from build123d import *

# Parameters (mm, degrees)
F1_DEPTH       = 30
F3_D           = 12.6
F3_CBORE_D     = 19.25
F3_CBORE_DEPTH = 12
F5_DEPTH       = 20
F7_DEPTH       = 10
F9_T1_DEPTH    = 80.6698729811
F9_T3_DEPTH    = 37.5
F9_T5_DEPTH    = 30
F9_T7_DEPTH    = 81.3397459622
F9_T9_DEPTH    = 40
F9_T12_ANGLE   = 90
F9_T14_ANGLE   = 90
F9_T16_ANGLE   = 117.3060073295
F9_T18_ANGLE   = 90
F9_T20_ANGLE   = 180
F9_T22_ANGLE   = 180
F10_DEPTH      = 20.001


# Not quite as in the source:
# - a fillet or chamfer that OpenCascade refuses, or shapes differently, is made with other operations: its cross-section is extruded or revolved along the edge and cut away or added


with BuildPart() as f1:
    # F0 (on Top) → F1 (new body)
    with BuildSketch(Plane.XY):
        with BuildLine():
            Line((0, -30), (0, 0))
            Line((0, 0), (30, 30))
            Line((30, 30), (40, 30))
            ThreePointArc((40, 30), (47.0710678119, 32.9289321881), (50, 40))
            Line((50, 40), (50, 50))
            ThreePointArc((50, 50), (47.0710678119, 57.0710678119), (40, 60))
            Line((40, 60), (-45, 60))
            ThreePointArc((-45, 60), (-48.6602540378, 56.3397459622), (-50, 51.3397459622))
            Line((-50, 51.3397459622), (-50, -30))
            ThreePointArc((-50, -30), (-47.0710678119, -37.0710678119), (-40, -40))
            Line((-40, -40), (-10, -40))
            ThreePointArc((-10, -40), (-2.9289321881, -37.0710678119), (0, -30))
        make_face()
    extrude(amount=F1_DEPTH)

    # F3 (through all)
    with Locations(Plane.XY.offset(30)):
        with Locations((35, 45)):
            CounterBoreHole(F3_D / 2, F3_CBORE_D / 2, F3_CBORE_DEPTH)

    # F4 (on face) → F5 (cut)
    with BuildSketch(Plane.XY.offset(30)):
        with BuildLine():
            Line((-10, 55.6698729811), (-42.5, 55.6698729811))
            ThreePointArc((-42.5, 55.6698729811), (-44.3301270189, 53.8397459622), (-45, 51.3397459622))
            Line((-45, 51.3397459622), (-45, -30))
            ThreePointArc((-45, -30), (-43.5355339059, -33.5355339059), (-40, -35))
            Line((-40, -35), (-10, -35))
            ThreePointArc((-10, -35), (-6.4644660941, -33.5355339059), (-5, -30))
            Line((-5, -30), (-5, 50.6698729811))
            ThreePointArc((-5, 50.6698729811), (-6.4644660941, 54.205406887), (-10, 55.6698729811))
        make_face()
    extrude(amount=-F5_DEPTH, mode=Mode.SUBTRACT)

    # F6 (on face) → F7 (join)
    with BuildSketch(Plane.XY.offset(10)):
        with BuildLine():
            ThreePointArc((-16.25, 30), (-26.25, 40), (-36.25, 30))
            Line((-36.25, 30), (-36.25, -10))
            ThreePointArc((-36.25, -10), (-26.25, -20), (-16.25, -10))
            Line((-16.25, -10), (-16.25, 30))
        make_face()
    extrude(amount=F7_DEPTH)

    # F9: fillet of radius 2 on 12 edges, made by hand

    # F9_s2 → F9_t1 (join)
    with BuildSketch(Plane.XZ.offset(-50.6698729811)):
        with BuildLine():
            ThreePointArc((-5, 12), (-5.5857864376, 10.5857864376), (-7, 10))
            Line((-7, 10), (-5, 10))
            Line((-5, 10), (-5, 12))
        make_face()
    extrude(amount=F9_T1_DEPTH)

    # F9_s4 → F9_t3 (join)
    with BuildSketch(Plane.YZ.offset(-47.5)):
        with BuildLine():
            ThreePointArc((55.6698729811, 12), (55.0840865435, 10.5857864376), (53.6698729811, 10))
            Line((53.6698729811, 10), (55.6698729811, 10))
            Line((55.6698729811, 10), (55.6698729811, 12))
        make_face()
    extrude(amount=F9_T3_DEPTH)

    # F9_s6 → F9_t5 (join)
    with BuildSketch(Plane.YZ.offset(-40)):
        with BuildLine():
            ThreePointArc((-35, 12), (-34.4142135624, 10.5857864376), (-33, 10))
            Line((-33, 10), (-35, 10))
            Line((-35, 10), (-35, 12))
        make_face()
    extrude(amount=F9_T5_DEPTH)

    # F9_s8 → F9_t7 (join)
    with BuildSketch(Plane.XZ.offset(-51.3397459622)):
        with BuildLine():
            ThreePointArc((-45, 12), (-44.4142135624, 10.5857864376), (-43, 10))
            Line((-43, 10), (-45, 10))
            Line((-45, 10), (-45, 12))
        make_face()
    extrude(amount=F9_T7_DEPTH)

    # F9_s10 → F9_t9 (join)
    with BuildSketch(Plane.XZ.offset(-30)):
        with BuildLine():
            ThreePointArc((-14.25, 10), (-15.6642135624, 10.5857864376), (-16.25, 12))
            Line((-16.25, 12), (-16.25, 10))
            Line((-16.25, 10), (-14.25, 10))
        make_face()
        with BuildLine():
            ThreePointArc((-38.25, 10), (-36.8357864376, 10.5857864376), (-36.25, 12))
            Line((-36.25, 12), (-36.25, 10))
            Line((-36.25, 10), (-38.25, 10))
        make_face()
    extrude(amount=F9_T9_DEPTH)

    # F9_s11 → F9_t12 (revolve)
    with BuildSketch(Plane.XZ.offset(-50.6698729811)):
        with BuildLine():
            ThreePointArc((-5, 12), (-5.5857864376, 10.5857864376), (-7, 10))
            Line((-7, 10), (-5, 10))
            Line((-5, 10), (-5, 12))
        make_face()
    revolve(axis=Axis((-10, 50.6698729811, 10), (0, 0, 1)), revolution_arc=F9_T12_ANGLE)

    # F9_s13 → F9_t14 (revolve)
    with BuildSketch(Plane.YZ.offset(-10)):
        with BuildLine():
            ThreePointArc((-35, 12), (-34.4142135624, 10.5857864376), (-33, 10))
            Line((-33, 10), (-35, 10))
            Line((-35, 10), (-35, 12))
        make_face()
    revolve(axis=Axis((-10, -30, 10), (0, 0, 1)), revolution_arc=F9_T14_ANGLE)

    # F9_s15 → F9_t16 (revolve)
    with BuildSketch(Plane(origin=(-52.509549327, 27.1091719145, 0), x_dir=(0, 0, 1), z_dir=(0.8885691394, -0.4587427214, 0))):
        with BuildLine():
            ThreePointArc((12, -32.2692050314), (10.5857864376, -31.6834185938), (10, -30.2692050314))
            Line((10, -30.2692050314), (10, -32.2692050314))
            Line((10, -32.2692050314), (12, -32.2692050314))
        make_face()
    revolve(axis=Axis((-40, 51.3397459622, 10), (0, 0, 1)), revolution_arc=F9_T16_ANGLE)

    # F9_s17 → F9_t18 (revolve)
    with BuildSketch(Plane.XZ.offset(30)):
        with BuildLine():
            ThreePointArc((-45, 12), (-44.4142135624, 10.5857864376), (-43, 10))
            Line((-43, 10), (-45, 10))
            Line((-45, 10), (-45, 12))
        make_face()
    revolve(axis=Axis((-40, -30, 10), (0, 0, 1)), revolution_arc=F9_T18_ANGLE)

    # F9_s19 → F9_t20 (revolve)
    with BuildSketch(Plane.XZ.offset(10)):
        with BuildLine():
            ThreePointArc((-38.25, 10), (-36.8357864376, 10.5857864376), (-36.25, 12))
            Line((-36.25, 12), (-36.25, 10))
            Line((-36.25, 10), (-38.25, 10))
        make_face()
    revolve(axis=Axis((-26.25, -10, 10), (0, 0, 1)), revolution_arc=F9_T20_ANGLE)

    # F9_s21 → F9_t22 (revolve)
    with BuildSketch(Plane.XZ.offset(-30)):
        with BuildLine():
            ThreePointArc((-14.25, 10), (-15.6642135624, 10.5857864376), (-16.25, 12))
            Line((-16.25, 12), (-16.25, 10))
            Line((-16.25, 10), (-14.25, 10))
        make_face()
    revolve(axis=Axis((-26.25, 30, 10), (0, 0, 1)), revolution_arc=F9_T22_ANGLE)

    # F8 (on face) → F10 (cut, through all)
    with BuildSketch(Plane.XY.offset(20)):
        with BuildLine():
            ThreePointArc((-31.25, -7.5), (-26.25, -12.5), (-21.25, -7.5))
            Line((-21.25, -7.5), (-21.25, 27.5))
            ThreePointArc((-21.25, 27.5), (-26.25, 32.5), (-31.25, 27.5))
            Line((-31.25, 27.5), (-31.25, -7.5))
        make_face()
    extrude(amount=-F10_DEPTH, mode=Mode.SUBTRACT)


solid = f1.part
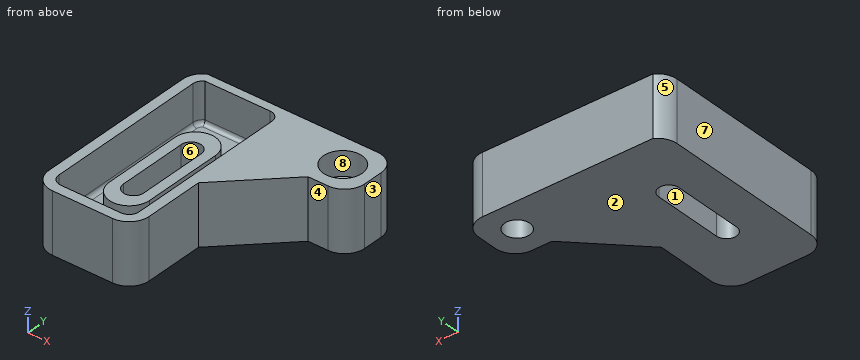
Can you work these out from the model? Positions are in its coordinate system, mm. Face numbers are marked on the shaded views. A direction names the side the tool comes from. Coordinates: 2 decimals unless noted, no trailing zeros. Order: outer loops, then holes, each group sorted by start corner. A loop starts at its lowest first (then second) coordinate and runs counter-clockwise, first axis right, second up. Notation, with made-up numbers: M 83.5,74 L 136.5,74 A28 ccw 136.5,108 Z; hole C -7,-19.75 d11. An arc over 180 degrees is marked long. Write item = value, one per line.
(1) Suppose I cut it at A-A on z = 13.5. State how many separate pieces and enclosed holes the cut face has, plus the area to 3 significant figures.
Results are:
separate_pieces = 2
enclosed_holes = 3
area = 3,800 mm2
(2) Suppose I cut it at C-C on y = 45. Please give me the cut outline in (x, z) (3 decimals), plus the area to 3 significant figures.
Results are:
outline = M -50,0 L 28.7,0 L 28.7,18 L 25.375,18 L 25.375,30 L -5,30 L -5,12 A2 cw -7,10 L -43,10 A2 cw -45,12 L -45,30 L -50,30 Z; M 41.3,0 L 50,0 L 50,30 L 44.625,30 L 44.625,18 L 41.3,18 Z
area = 1,740 mm2
(3) For pin 1 Ø6 at (y, z) = (4, 25) entering from +X; pin 2 Ø11.5 at (x, y) = (35, 45) entering from -Z (3 decimals); pin 3 Ø9 at (y, z) = (5.5, 21) entering from +X; pin 4 Ø11 at (x, y) = (-31.5, -11) entering from +Z, each with a flat end and sliding along its axis, tell me the tip position at first contact or that it passes through.
Results are:
pin_1 = 7
pin_2 = through
pin_3 = 10
pin_4 = 20
(4) If we mould it in two halves opening along X, with no side actions, what happens to the marked faces 1, 2 and 3? For each: pulls with the +X half, pulls with the -X half, needs draft (parallel to the pull), parting line crosses it, or undercut.
Results are:
face_1 = undercut
face_2 = needs draft
face_3 = pulls with the +X half
(5) I need wall thicknesses on line 1 along X through (y, z) = (-15.5, 29); line 2 along Y through (x, z) = (-10, 21.75); line 3 along Y through (x, z) = (35, 13.5). Which ranges of each line are inside material? Lowest first, please. Write a range as [from, to].
Results are:
line_1 = [-50, -45], [-5, 0]
line_2 = [-40, -35], [55.67, 60]
line_3 = [30, 38.7], [51.3, 60]
(6) Suppose I cut it at D-D on z = 4.5. Please give me the cut outline in (x, y).
Results are:
outline = M -50,-30 A10 ccw -40,-40 L -10,-40 A10 ccw 0,-30 L 0,0 L 30,30 L 40,30 A10 ccw 50,40 L 50,50 A10 ccw 40,60 L -45,60 A10 ccw -50,51.34 Z; hole M -31.25,-7.5 A5 ccw -21.25,-7.5 L -21.25,27.5 A5 ccw -31.25,27.5 Z; hole C 35,45 d12.6
(7) Suppose I cut it at B-B on x = -26.25. Please give me the cut outline in (y, z).
Results are:
outline = M -40,0 L -12.5,0 L -12.5,20 L -20,20 L -20,12 A2 cw -22,10 L -33,10 A2 cw -35,12 L -35,30 L -40,30 Z; M 32.5,0 L 60,0 L 60,30 L 55.67,30 L 55.67,12 A2 cw 53.67,10 L 42,10 A2 cw 40,12 L 40,20 L 32.5,20 Z
(8) For the marked faces 4, 5, 6, 7 and 8, which set-ups out of +Z, -Z, +X, -X, +Y, -Y let a thin tool reach every point of the face, with its end or its side?
Results are:
face_4 = +Z, -Z, +X, -Y
face_5 = +Z, -Z, -X, +Y
face_6 = +Z, -Z
face_7 = +Z, -Z, -X, +Y, -Y
face_8 = +Z
